```python
from build123d import *

# Parameters (mm, degrees)
F0_W     = 60
F0_H     = 25
F1_DEPTH = 5.5
F2_R     = 3


with BuildPart() as f1:
    # F0 (on Top) → F1 (new body)
    with BuildSketch(Plane.XY):
        with Locations((30, -12.5)):
            Rectangle(F0_W, F0_H)
        with BuildLine():
            ThreePointArc((32.142429, -10.225), (30, -15.625), (27.857571, -10.225))
            Line((27.857571, -10.225), (32.142429, -10.225))
        make_face(mode=Mode.SUBTRACT)
    extrude(amount=F1_DEPTH)

    # F2
    f2_edges = [f1.edges().sort_by_distance(p)[0] for p in [
        (0, -25, 2.75),
        (60, -25, 2.75),
        (60, 0, 2.75),
        (0, 0, 2.75),
    ]]
    fillet(f2_edges, radius=F2_R)


solid = f1.part
```
Model file for the job. Use its own axes, mm. Round coordinates to 2 decimals unless told otherwise and drop trailing zeros. Loops run counter-clockwise (first coordinate to the right, second up) from the corner with the lowest first, then second, coordinate; pieces in that order, holes last. Notation, with made-up numbers: M 73.25,72 L 87.25,72 A8 cw 87.25,85 Z; hole C -18.5,42 d2. An arc over 180 degrees is marked long. Put each result on its own line as item: value. Start each with the question number.
Item 1: Drill centre lines: line 1 along Y through (x, z) = (30, 2.9) (3 decimals); line 2 along X through (y, z) = (-12.5, 3.6) (3 decimals); line 3 along X through (y, z) = (-13.5, 3.5). Where is each one in solid material? Low to high.
Item 2: Cut at B-B (y = -12.5). List the corners of the cut face in (x, z) (3 decimals).
Item 3: Cut at A-A (x = 30). List the corners of the cut face in (y, z) (3 decimals).
Item 4: Cut at C-C (z = 3.7). List the corners of the cut face in (x, y) (3 decimals), then the cut area to 3 significant figures.
Item 5: Mould opens along X. For faces 1 (the face through (0.86, -24.1, 2.79)), 2 (the face through (60, -13, 3)), 3 (the face through (30, -10.225, 3)) say: released by +X, released by -X, zero draft, split by the parting line, or undercut.
Answer block:
1. line 1: -25 to -15.625, -10.225 to 0
1. line 2: 0 to 26.875, 33.125 to 60
1. line 3: 0 to 27.04, 32.96 to 60
2. outline: M 0,0 L 26.875,0 L 26.875,5.5 L 0,5.5 Z; M 33.125,0 L 60,0 L 60,5.5 L 33.125,5.5 Z
3. outline: M -25,0 L -15.625,0 L -15.625,5.5 L -25,5.5 Z; M -10.225,0 L 0,0 L 0,5.5 L -10.225,5.5 Z
4. outline: M 0,-22 A3 ccw 3,-25 L 57,-25 A3 ccw 60,-22 L 60,-3 A3 ccw 57,0 L 3,0 A3 ccw 0,-3 Z; hole M 27.858,-10.225 A3.125 ccw long 32.142,-10.225 Z
4. area: 1,460 mm2
5. face 1: released by -X
5. face 2: released by +X
5. face 3: undercut
